Design review of the part built by this model. Coordinates are the model's own, in mm. Face numbers are marked on the shaded views. A direction names the side the tool comes from. Coordinates: 2 decimals unless noted, no trailing zeros. Write each loop counter-clockwise with the first axis right and the second up, starting at its lowest first coordinate (ties: lowest second). Pieces come first, ordered by that corner, then holes.
Q1. For probe 1 along Y at (x, z) = (0, 5) (3 decimals); probe 2 along X at (y, z) = (-2, 2.5); probe 3 along Z at (x, y) = (6.75, 8), list the stretches that pass through material, from the lowest coordinate up.
Q2. Take a section at D-D (z = 10.75). Give the boundary of the cut face in (x, y) (3 decimals), and give its area (3 significant figures).
Q3. Insertion check: pin 1 (8 mm diameter, centred on x = 2, z = 2, fed in from +Y) (3 decimals); pin 2 (3 mm diameter, centred on x = -6, z = 2.5, fed in from -Y). Each pin has a flat end and moves straight along its axis. Give the tip position at first contact, or say it passes through.
Q4. Machinability: for the marked faces 1 and 2, which of the approach directions +Z, -Z, +X, -X, +Y, -Y give a long, thin tool a straight path to every point of the face, cutting with its end or side? Answer none if there is none.
Q5. Take a section at B-B (z = 3.25). Give the boundary of the cut face in (x, y) (3 decimals).
Autodesk Inventor part; units mm, degrees
ref_plane "YZ Plane" through (0, 0, 0) normal (1, 0, 0) x (0, 1, 0)
ref_plane "XZ Plane" through (0, 0, 0) normal (0, 1, 0) x (-1, 0, 0)
ref_plane "XY Plane" through (0, 0, 0) normal (0, 0, 1) x (1, 0, 0)
sketch "Sketch1" plane through (0, 0, 0) normal (0, 0, 1) x (1, 0, 0)
  circle A0 centre (0, 0) radius 1.7
  circle A1 centre (0, 0) radius 2.2
  circle A2 centre (0, 0) radius 3.375
  dimension "d0" = 3.4
  dimension "d1" = 0.5
  dimension "d3" = 6.75
extrude "Extrusion1" add sketch "Sketch1" along normal blind 10
sketch "Sketch2" plane through (0, 0, 10) normal (0, 0, 1) x (1, 0, 0)
  circle A0 centre (0, 0) radius 3.375
  dimension "d6" = 6.75
extrude "Extrusion2" add sketch "Sketch2" along normal blind 6
sketch "Sketch3" plane through (0, 0, 16) normal (0, 0, 1) x (1, 0, 0)
  circle A0 centre (0, 0) radius 12.5
  dimension "d12" = 25
extrude "Extrusion3" add sketch "Sketch3" along normal blind 0.5
chamfer "Chamfer2" distance 9.125 distance2 4 1 edges at (-3.375, 0, 16) measured on face at (9.3373, -0.9971, 16)
properties part number "SpringCapV1"
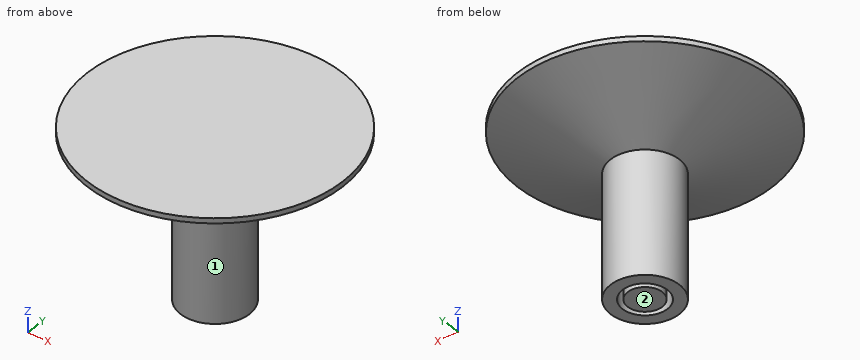
Response:
1. probe 1: y = -3.375 to -2.2, -1.7 to 1.7, 2.2 to 3.375
1. probe 2: x = -2.72 to -0.92, 0.92 to 2.72
1. probe 3: z = 15.11 to 16.5
2. outline: circle Ø6.75 at (0, 0)
2. area: 35.8 mm2
3. pin 1: stops at y = 3.375
3. pin 2: passes through
4. face 1: -Z
4. face 2: -Z, +X, -X, +Y, -Y
5. outline: circle Ø6.75 at (0, 0); circle Ø3.4 at (0, 0); hole circle Ø4.4 at (0, 0)
